from build123d import *

# Parameters (mm, degrees)
SKETCH1_W           = 20
SKETCH1_H           = 20
SKETCH1_R           = 8
FIRSTLAYER_DEPTH    = 5
SKETCH2_W           = 20
SKETCH2_H           = 20
SKETCH2_R           = 6
SECONDLAYER_DEPTH   = 0.5
SKETCH3_W           = 20
SKETCH3_H           = 20
THIRDLAYER_DEPTH    = 5.5
SKETCH4_W           = 20
SKETCH4_H           = 11
BOSS_EXTRUDE4_DEPTH = 10
SKETCH10_W          = 5.42
SKETCH10_H          = 2.36
NUT_HOLE_DEPTH      = 5.5
NUT_HOLE_DEPTH_BACK = 2.71
SKETCH11_R          = 1.5
SCREW_HOLE_DEPTH    = 5.64


with BuildPart() as part:
    # Sketch1 → FirstLayer (new body)
    with BuildSketch(Plane.XY):
        Rectangle(SKETCH1_W, SKETCH1_H)
        Circle(SKETCH1_R, mode=Mode.SUBTRACT)
    extrude(amount=-FIRSTLAYER_DEPTH)

    # Sketch2 → SecondLayer (add)
    with BuildSketch(Plane.XY):
        Rectangle(SKETCH2_W, SKETCH2_H)
        Circle(SKETCH2_R, mode=Mode.SUBTRACT)
    extrude(amount=SECONDLAYER_DEPTH)

    # Sketch3 → ThirdLayer (add)
    with BuildSketch(Plane.XY.offset(0.5)):
        Rectangle(SKETCH3_W, SKETCH3_H)
    extrude(amount=THIRDLAYER_DEPTH)

    # Sketch4 → Boss-Extrude4 (add)
    with BuildSketch(Plane(origin=(0, 10, 0), x_dir=(1, 0, 0), z_dir=(0, 1, 0))):
        with Locations((0, -0.5)):
            Rectangle(SKETCH4_W, SKETCH4_H)
    extrude(amount=BOSS_EXTRUDE4_DEPTH)

    # Sketch10 → Nut Hole (cut, two sides)
    with BuildSketch(Plane(origin=(0, 0, 0.5), x_dir=(-1, 0, 0), z_dir=(0, 0, -1))) as nut_hole_sk:
        with Locations((0, 13.18)):
            Rectangle(SKETCH10_W, SKETCH10_H)
    extrude(amount=NUT_HOLE_DEPTH, mode=Mode.SUBTRACT)
    extrude(nut_hole_sk.sketch, amount=-NUT_HOLE_DEPTH_BACK, mode=Mode.SUBTRACT)

    # Sketch11 → Screw Hole (cut)
    with BuildSketch(Plane(origin=(0, 20, 0), x_dir=(1, 0, 0), z_dir=(0, 1, 0))):
        with Locations((0, -0.5)):
            Circle(SKETCH11_R)
    extrude(amount=-SCREW_HOLE_DEPTH, mode=Mode.SUBTRACT)


solid = part.part
Could you check a few things on this model? Use its own coordinates, in mm. A direction names the side the tool comes from. Give positions to 0.01 mm unless a question says otherwise; leave off trailing zeros. Order: outer loops, then holes, each group sorted by start corner. A loop starts at its lowest first (then second) coordinate and runs counter-clockwise, first axis right, second up. Notation, with made-up numbers: (20, -31) - (40, -31) arc R8 ccw to (40, -21) - close; hole circle Ø9 at (46.25, 61). An arc over 180 degrees is marked (long way). One line per question, with ' | ' between items. Start each with the question number.
Item 1: I want a section at B-B on z = 2.75. Write out the boundary of the cut face in (x, y), then the cut area to 3 significant figures.
Item 2: I want a section at D-D on z = -1.5. Write out the boundary of the cut face in (x, y).
Item 3: I want a section at C-C on y = 18. Write out the boundary of the cut face in (x, z), then the cut area to 3 significant figures.
Item 4: Thinking about a two-plate mould opening in X: for faces 4 (the flat face through (10, 5, 1)), 5 (the flat face through (0, 5, 6)), 6 (the flat face through (0, 0, 0.5)), which applies, pulls with the +X half, pulls with the -X half, needs draft (parallel to the pull), parting line crosses it, or undercut?
Item 5: I want a section at A-A on x = 0. Write out the boundary of the cut face in (y, z), then the cut area to 3 significant figures.
Item 6: I need wall thicknesses on probe 1 along Y at (x, z) = (0, -2.8); probe 2 along Y at (x, z) = (1.75, 2.25); probe 3 along Y at (x, z) = (0, 0.25). Which ranges of each line are inside material? Lowest first, please. Write a range as [from, to].
Item 7: I'm going to push flat-ended pins straight in: pin 1 Ø9.5 at (x, y) = (0, 0) entering from -Z; pin 2 Ø6 at (x, y) = (-2, 3) entering from -Z; pin 3 Ø0.7 at (x, y) = (0, 13) entering from -Z. Where does each tip first touch, or does it pass through?
Item 8: For faces 1 (the cylindrical face through (0, 17, 2)), 2 (the cylindrical face through (-5.994, 0.264, 0.246)), 3 (the flat face through (2, 8, -5)), which set-ups out of +Z, -Z, +X, -X, +Y, -Y let a thin tool reach every point of the face, with its end or its side?
Verdict:
1) outline: (-10, -10) - (10, -10) - (10, 20) - (-10, 20) - close; hole (-2.71, 12) - (2.71, 12) - (2.71, 14.36) - (-2.71, 14.36) - close | area: 587 mm^2
2) outline: (-10, -10) - (10, -10) - (10, 20) - (-10, 20) - close; hole circle Ø16 at (0, 0); hole (-2.71, 12) - (2.71, 12) - (2.71, 14.36) - (-2.71, 14.36) - close
3) outline: (-10, -5) - (10, -5) - (10, 6) - (-10, 6) - close; hole circle Ø3 at (0, 0.5) | area: 213 mm^2
4) face 4: pulls with the +X half | face 5: needs draft | face 6: undercut
5) outline: (-10, -5) - (-8, -5) - (-8, 0) - (-6, 0) - (-6, 0.5) - (6, 0.5) - (6, 0) - (8, 0) - (8, -5) - (12, -5) - (12, 3.21) - (14.36, 3.21) - (14.36, 2) - (20, 2) - (20, 6) - (-10, 6) - close; (14.36, -5) - (20, -5) - (20, -1) - (14.36, -1) - close | area: 208 mm^2
6) probe 1: [-10, -8], [8, 12], [14.36, 20] | probe 2: [-10, 12], [14.36, 20] | probe 3: [-10, -6], [6, 12]
7) pin 1: z = 0.5 | pin 2: z = 0 | pin 3: z = 3.21
8) face 1: +Y | face 2: -Z | face 3: -Z, +X, -X, +Y, -Y
